Source: CAD feature listing. Evaluate the final solid. Frame: model axes, mm. Face numbers are marked on the shaded views. A direction names the side the tool comes from. Give positions to 0.01 mm unless a question says otherwise; leave off trailing zeros. Order: outer loops, then holes, each group sorted by start corner. A loop starts at its lowest first (then second) coordinate and runs counter-clockwise, first axis right, second up.
from build123d import *

# Parameters (mm, degrees)
EXTRUDE1_DEPTH     = 152.4
SKETCH2_R          = 3.175
CUT_EXTRUDE1_DEPTH = 446.134547075


with BuildPart() as part:
    # Sketch1 → Extrude1 (new, symmetric)
    with BuildSketch(Plane.XY):
        with BuildLine():
            Line((323.85, 6.35), (323.85, -6.35))
            Line((323.85, -6.35), (17.960512242, -6.35))
            ThreePointArc((17.960512242, -6.35), (-19.05, 0), (17.960512242, 6.35))
            Line((17.960512242, 6.35), (323.85, 6.35))
        make_face()
    extrude(amount=EXTRUDE1_DEPTH, both=True)

    # Sketch2 → Cut-Extrude1 (cut, through all)
    with BuildSketch(Plane.XY.offset(152.4)):
        with Locations((63.5, 0)):
            Circle(SKETCH2_R)
    extrude(amount=-CUT_EXTRUDE1_DEPTH, mode=Mode.SUBTRACT)


solid = part.part
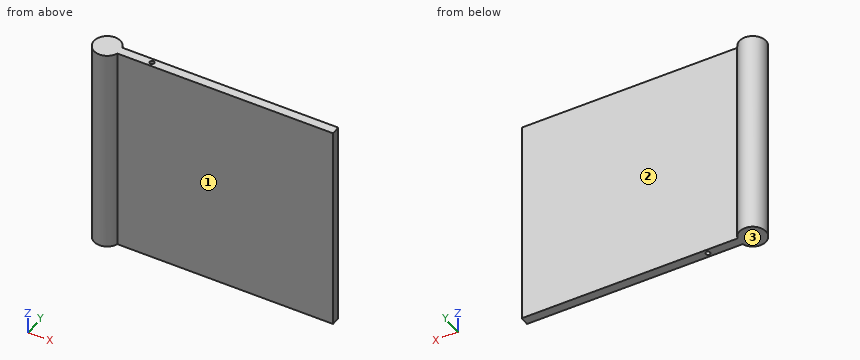
1) First-contact query: pin 1 Ø10 at (x, z) = (221.5, -98.5) entering from -Y; pin 2 Ø5 at (y, z) = (-9, -11) entering from -X; pin 3 Ø6 at (x, z) = (196, 17) entering from +Y. Flat tips, straight axial feed; report the tip coordinate or a pass-through.
Checks:
pin 1: stops at y = -6.35
pin 2: stops at x = -17.91
pin 3: stops at y = 6.35
2) Section query A-A on z = -129. Output: boundary loops of the cut face in (x, y) (3 decimals).
Checks:
outline: (17.961, -6.35) - (323.85, -6.35) - (323.85, 6.35) - (17.961, 6.35) arc R19.05 ccw (long way) to start; hole circle Ø6.35 at (63.5, 0)
3) Ray query, L1, parallel to Y at x = 63.5, z = -22 (3 decimals); L2, parallel to Y at x = 63, z = -60; L3, parallel to Y at x = 104.5, z = 134. Return the intervals inside material, ascending.
Checks:
L1: y = -6.35 to -3.175, 3.175 to 6.35
L2: y = -6.35 to -3.14, 3.14 to 6.35
L3: y = -6.35 to 6.35
4) Section query B-B on x = 165. Output: boundary loops of the cut face in (y, z), and give its area (3 significant figures).
Checks:
outline: (-6.35, -152.4) - (6.35, -152.4) - (6.35, 152.4) - (-6.35, 152.4) - close
area: 3,870 mm2
5) Reachability of the marked faces 1, 2 and 3 from +Z, -Z, +X, -X, +Y, -Y: full face, straight path, thin tool, end or side. Return the list, or none.
Checks:
face 1: +Z, -Z, +X, -Y
face 2: +Z, -Z, +X, +Y
face 3: -Z, +X, -X, +Y, -Y
